CAD build for the part. Positions are in the model's coordinates, mm. A direction names the side the tool comes from. Round coordinates to 2 decimals unless told otherwise and drop trailing zeros. Order: outer loops, then holes, each group sorted by start corner. A loop starts at its lowest first (then second) coordinate and runs counter-clockwise, first axis right, second up. Notation, with made-up numbers: M -37.5,57 L -0.5,57 A25 cw -0.5,70 Z; hole C -6,51.25 d10. An arc over 180 degrees is marked long. Answer as a JSON object with one key per item and string values. Group by question number.
```python
from build123d import *

# Parameters (mm, degrees)
SKETCH1_R           = 10
SKETCH1_R_2         = 7.5
BOSS_EXTRUDE1_DEPTH = 20
SKETCH2_R           = 10
BOSS_EXTRUDE2_DEPTH = 2.5
SKETCH3_R           = 6
CUT_EXTRUDE1_DEPTH  = 2.5
FILLET1_R           = 1


with BuildPart() as part:
    # Sketch1 → Boss-Extrude1 (new body)
    with BuildSketch(Plane.XY):
        Circle(SKETCH1_R)
        Circle(SKETCH1_R_2, mode=Mode.SUBTRACT)
    extrude(amount=BOSS_EXTRUDE1_DEPTH)

    # Sketch2 → Boss-Extrude2 (add)
    with BuildSketch(Plane.XY.offset(20)):
        Circle(SKETCH2_R)
    extrude(amount=BOSS_EXTRUDE2_DEPTH)

    # Sketch3 → Cut-Extrude1 (cut)
    with BuildSketch(Plane.XY.offset(22.5)):
        Circle(SKETCH3_R)
    extrude(amount=-CUT_EXTRUDE1_DEPTH, mode=Mode.SUBTRACT)

    # Fillet1
    fillet1_edges = [part.edges().sort_by_distance(p)[0] for p in [
        (-10, 0, 22.5),
    ]]
    fillet(fillet1_edges, radius=FILLET1_R)


solid = part.part
```
Item 1: Cut at A-A, the plane y = 0. Give the cut face in (x, z), and give its area (3 significant figures).
Item 2: Drill centre lines: line 1 (Y direction, x = 0, z = 9.5); line 2 (Z direction, x = 7, y = -1.25); line 3 (Z direction, x = 7.25, y = -5.5). Where is each one in solid material? Low to high. Write a range as [from, to].
Item 3: Two-plate mould, pull along X, no slides. Class faces 1 (the face through (-2.17, -9.76, 10.6)), 2 (the face through (2, 6, 20)), 3 (the face through (2, -6, 22.5)): +X half, -X half, draft (parallel to the pull), parting line (faces both ways), or undercut.
Item 4: Flat gauge pins, fed straight in: pin 1 Ø3 at (x, z) = (3.5, 11) entering from +Y; pin 2 Ø10 at (x, z) = (-5.5, 19.5) entering from +Y; pin 3 Ø9.5 at (x, y) = (0, 0) entering from +Z; pin 4 Ø1.5 at (y, z) = (6.5, 10) entering from -X. Where does each tip first touch, or does it go through?
Item 5: Cut at C-C, the plane z = 17.5. Give the cut face in (x, y), and give its area (3 significant figures).
Item 6: 3-axis set-ups, long thin cutter, end or side, ignore diameter. For faces 4 (the face through (-6, 0, 21)), 5 (the face through (-7.493, 0.33, 9.86)): which of +Z, -Z, +X, -X, +Y, -Y reach the whole face in a straight line?
Response values:
{
 "1": {"outline": "M -10,0 L -7.5,0 L -7.5,20 L -6,20 L -6,22.5 L -9,22.5 A1 ccw -10,21.5 Z; M 6,20 L 7.5,20 L 7.5,0 L 10,0 L 10,21.5 A1 ccw 9,22.5 L 6,22.5 Z", "area": "120 mm^2"},
 "2": {"line 1": "[-10, -7.5], [7.5, 10]", "line 2": "[20, 22.5]", "line 3": "[0, 22.49]"},
 "3": {"face 1": "parting line", "face 2": "undercut", "face 3": "draft"},
 "4": {"pin 1": "y = 9.8", "pin 2": "y = 9.99", "pin 3": "through", "pin 4": "x = -8.18"},
 "5": {"outline": "C 0,0 d20; hole C 0,0 d15", "area": "137 mm^2"},
 "6": {"face 4": "+Z, -Z", "face 5": "-Z"}
}
